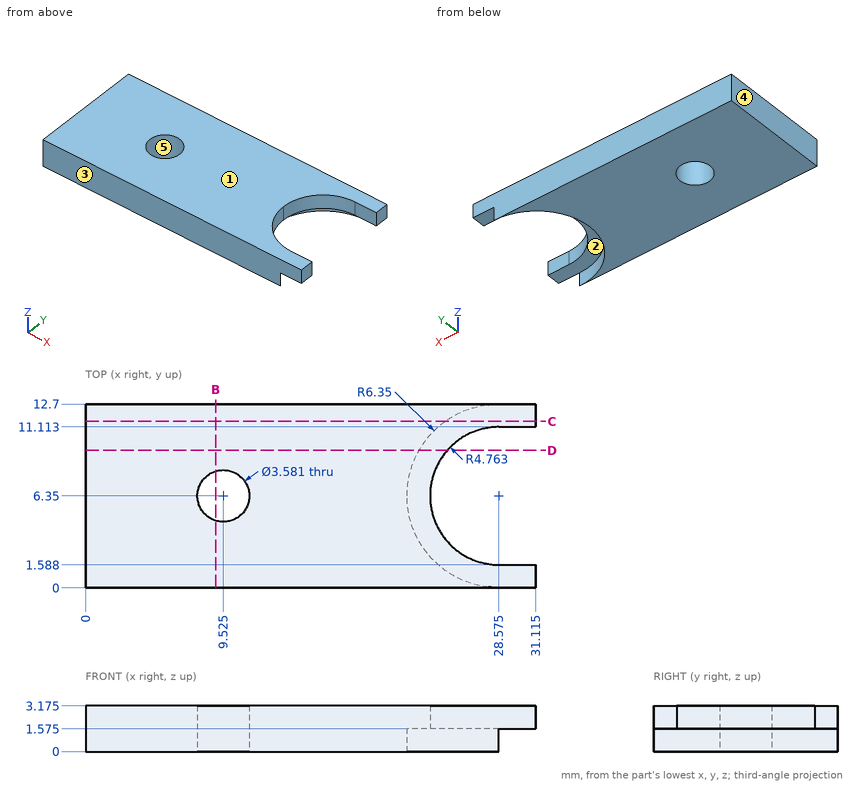
Study the drawing (mm; zero at the part's minimum x, y, z) and answer. A direction names the side the tool comes from. Give positions to 0.01 mm unless a question says otherwise; leave off trailing zeros. Write each loop counter-clockwise with the first axis right and the second up, starting at its lowest first coordinate (ties: lowest second). Pieces come first, ordered by that corner, then holes. Notation, with made-up numbers: (-22, -8) -> (1, -8) arc R14 ccw to (1, 1) -> close; hole circle Ø4 at (83.5, 46.25). An arc over 180 degrees is marked (long way). Write item = value, one per line. Start each with the question number.
1) Which of the six approach directions +Z, -Z, +X, -X, +Y, -Y give full straight-line access (tool end or side, diameter ignored) to the marked faces 1 and 2?
2) This flat-tipped pin is pushed along its axis until it touches: pin 1 (4.5 mm diameter, centred on x = 9.525, y = 6.35, fed in from -Z). Where does it stop, or does it pass through?
3) Determine the mould class of the marked faces 3, 4 and 5 for opening direction X: +X half, -X half, draft (parallel to the pull), parting line (faces both ways), or undercut.
4) Straight lines are drawn through the part: line 1 along Y through (x, z) = (27, 0.95); line 2 along X through (y, z) = (7, 2.1) (1 decimal); line 3 along Z through (x, y) = (24, 2.25) (1 decimal). For each, find the intervals that lie inside material, in ascending order.
5) The part is cut by section D-D, the plane y = 9.5. Determine the outline of the cut face in (x, z) (1 decimal).
6) The part is cut by section C-C, the plane y = 11.5. Determine the outline of the cut face in (x, z) (1 decimal).
7) The part is cut by section B-B, the plane x = 9. Determine the outline of the cut face in (y, z) (1 decimal).
Solutions:
q1.face_1 = +Z, +X, -X, +Y, -Y
q1.face_2 = -Z, +X
q2.pin_1 = 0
q3.face_3 = draft
q3.face_4 = -X half
q3.face_5 = undercut
q4.line_1 = 0 to 0.2, 12.5 to 12.7
q4.line_2 = 0 to 7.9, 11.2 to 23.9
q4.line_3 = 1.6 to 3.2
q5.outline = (0, 0) -> (23.1, 0) -> (23.1, 1.6) -> (25, 1.6) -> (25, 3.2) -> (0, 3.2) -> close
q6.outline = (0, 0) -> (24.9, 0) -> (24.9, 1.6) -> (31.1, 1.6) -> (31.1, 3.2) -> (0, 3.2) -> close
q7.outline = (0, 0) -> (4.6, 0) -> (4.6, 3.2) -> (0, 3.2) -> close; (8.1, 0) -> (12.7, 0) -> (12.7, 3.2) -> (8.1, 3.2) -> close
